from build123d import *

# Parameters (mm, degrees)
F0_W     = 304.8
F0_H     = 101.6
F0_R     = 6.7437
F1_DEPTH = 12.7
F2_R     = 7.9375
F3_DEPTH = 25.4


with BuildPart() as f1:
    # F0 (on Top) → F1 (new body)
    with BuildSketch(Plane.XY):
        with Locations((152.4, 50.8)):
            Rectangle(F0_W, F0_H)
        with Locations((69.85, 25.4)):
            Circle(F0_R, mode=Mode.SUBTRACT)
        with Locations((234.95, 25.4)):
            Circle(F0_R, mode=Mode.SUBTRACT)
        with Locations((69.85, 76.2)):
            Circle(F0_R, mode=Mode.SUBTRACT)
        with Locations((234.95, 76.2)):
            Circle(F0_R, mode=Mode.SUBTRACT)
    extrude(amount=F1_DEPTH)

    # F2 (on face) → F3 (cut)
    with BuildSketch(Plane(origin=(0, 0, 0), x_dir=(1, 0, 0), z_dir=(0, 0, -1))):
        with Locations((152.4, -50.8)):
            Circle(F2_R)
    extrude(amount=-F3_DEPTH, mode=Mode.SUBTRACT)


solid = f1.part
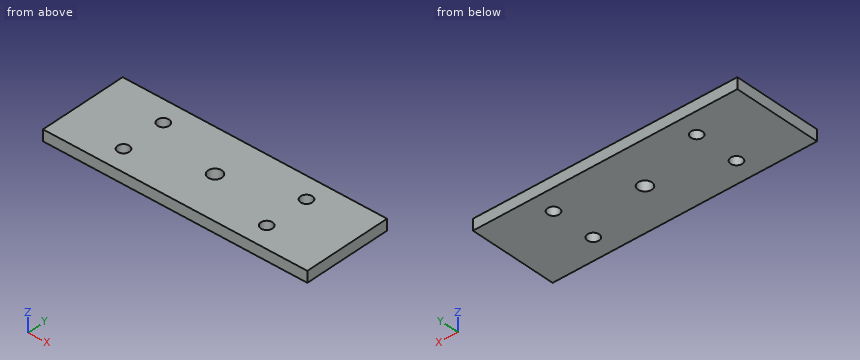
Design review of the part built by this model. Coordinates are the model's own, in mm. Round coordinates to 2 decimals unless told otherwise and drop trailing zeros. Write each loop counter-clockwise with the first axis right and the second up, starting at its lowest first coordinate (ties: lowest second). Pieces come first, ordered by that corner, then holes.
Item 1: Consider section B-B on z = 10. Count the separate pieces of the cut face and the enclosed holes in it, and give its area (3 significant figures).
Item 2: Consider section D-D on y = 46. Give the boundary of the cut face in (x, z), and give its area (3 significant figures).
Item 3: For pin 1 Ø2 at (x, y) = (160.5, 61) entering from -Z, flat-tipped, find the tip position at first contact; note if it passes through.
Item 4: Consider section A-A on x = 152.4. Give the boundary of the cut face in (y, z).
Item 5: Consider section C-C on y = 76.2. Give the boundary of the cut face in (x, z), and give its area (3 significant figures).
Item 6: Wall thickness on L1, parallel to Y at x = 69.85, z = 6.25; L2, parallel to Y at x = 152.4, z = 5; L3, parallel to X at y = 50.8, z = 10.25: over which ranges is each line inside the solid? List them lowest first.
Check values:
1. separate pieces: 1
1. enclosed holes: 5
1. area: 30,200 mm2
2. outline: (0, 0) - (146.08, 0) - (146.08, 12.7) - (0, 12.7) - close; (158.72, 0) - (304.8, 0) - (304.8, 12.7) - (158.72, 12.7) - close
2. area: 3,710 mm2
3. pin 1: stops at z = 0
4. outline: (0, 0) - (42.86, 0) - (42.86, 12.7) - (0, 12.7) - close; (58.74, 0) - (101.6, 0) - (101.6, 12.7) - (58.74, 12.7) - close
5. outline: (0, 0) - (63.11, 0) - (63.11, 12.7) - (0, 12.7) - close; (76.59, 0) - (228.21, 0) - (228.21, 12.7) - (76.59, 12.7) - close; (241.69, 0) - (304.8, 0) - (304.8, 12.7) - (241.69, 12.7) - close
5. area: 3,530 mm2
6. L1: y = 0 to 18.66, 32.14 to 69.46, 82.94 to 101.6
6. L2: y = 0 to 42.86, 58.74 to 101.6
6. L3: x = 0 to 144.46, 160.34 to 304.8
